Autodesk Inventor part; units mm, degrees
ref_plane "Start Plane" through (0, 0, -4.9897) normal (0, 0, 1) x (1, 0, 0)
ref_plane "End Plane" through (0, 0, 105.0166) normal (0, 0, 1) x (1, 0, 0)
ref_plane "Work Plane4" through (-9.4897, 4.8737, -6.8509) normal (0.4807, -0.2469, -0.8414) x (-0.4571, 0.7483, -0.4807)
ref_plane "Start Plane" through (0, 0, -4.9897) normal (0, 0, 1) x (1, 0, 0)
ref_plane "End Plane" through (0, 0, 105.0166) normal (0, 0, 1) x (1, 0, 0)
sketch "Sketch" plane through (0, 0, 0) normal (0, 0, 1) x (1, 0, 0)
  circle A0 centre (0, 0) radius 6.9342
  circle A1 centre (0, 0) radius 10.668
  dimension "d0" = 21.336
  dimension "d1" = 3.7338
extrude "Body" add sketch "Sketch" along normal up to surface (110.0063 mm away) from surface at -4.9897
sketch "Sketch3" plane through (0, 0, 0) normal (0, 0, 1) x (1, 0, 0)
  line L0 (0, 0) -> (10, 0)
ref_plane "Work Plane3" through (0, 0, 0) normal (0, -1, 0) x (1, 0, 0)
sketch "Sketch4" plane through (0, 0, 0) normal (0, -1, 0) x (1, 0, 0)
  line L0 (-2, -4.9897) -> (12, -4.9897)
  line L1 (-2, 105.0166) -> (12, 105.0166)
  dimension "d7" = 110.0063
ref_plane "Work Plane4" through (-9.4897, 4.8737, -6.8509) normal (0.4807, -0.2469, -0.8414) x (-0.4571, 0.7483, -0.4807)
split "Split1" plane through (-9.4897, 4.8737, -6.8509) removes the side toward (0.4807, -0.2469, -0.8414)
ref_plane "Work Plane5" through (6.4449, 8.5011, -9.0952) normal (-0.392, -0.517, -0.761) x (0.3573, -0.8478, 0.392)
split "Split2" plane through (6.4449, 8.5011, -9.0952) removes the side toward (-0.392, -0.517, -0.761)
ref_plane "Work Plane6" through (-10.5607, 1.5089, 115.9586) normal (0.7772, -0.111, 0.6194) x (0.627, 0.0533, -0.7772)
split "Split3" plane through (-10.5607, 1.5089, 115.9586) removes the side toward (0.7772, -0.111, 0.6194)
ref_plane "Work Plane7" through (0, 10.668, 105.0198) normal (0, -0.2353, 0.9719) x (1, 0, 0)
split "Split4" plane through (0, 10.668, 105.0198) removes the side toward (0, -0.2353, 0.9719)
equation "\"d0\" = G_H"
equation "\"d1\" = G_T"
equation "\"d2\" = G_L"
equation "\"G_H\" = 21.336"
equation "\"G_T\" = 3.7338"
equation "\"G_L\" = 110.00626"
equation "\"G_OFFSET_START\" = 4.98966"
equation "\"G_OFFSET_END\" = 2.57893"
equation "\"d4\" = -G_OFFSET_START"
equation "\"d5\" = G_OFFSET_END + B_L"
equation "\"B_L\" = 102.43767"
properties part number "ANSI - 1/2 x 0.147 - 4.331" material "Steel, Mild"
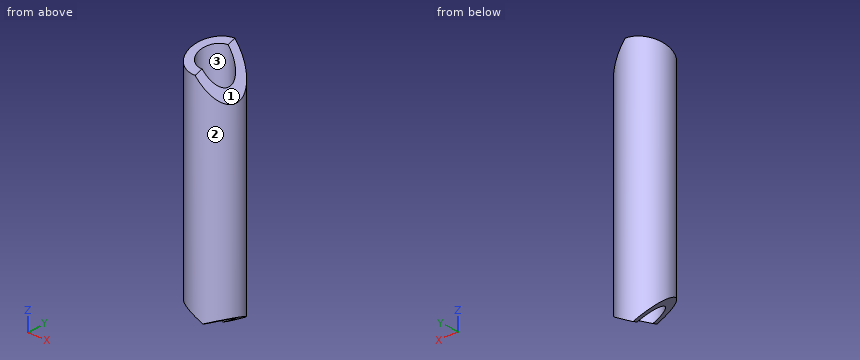
Geometry check sheet. Reference: the model listing, model coordinates, mm. Face numbers are marked on the shaded views. Round coordinates to 2 decimals unless told otherwise and drop trailing zeros. Loops run counter-clockwise (first coordinate to the right, second up) from the corner with the lowest first, then second, coordinate; pieces in that order, holes last.
Item 1: Cross-section at B-B on z = 85. Record the boundary of the cut face in (x, y), then the cut area to 3 significant figures.
Item 2: Cross-section at A-A on y = 2.5. Record the boundary of the cut face in (x, z), then the cut area to 3 significant figures.
Item 3: Cross-section at C-C on y = -5.5. Record the boundary of the cut face in (x, z).
Item 4: Gauge pin test, flat ends, axial feed: pin 1 (4 mm diameter, centred on y = -3, z = 90, fed in from -X); pin 2 (1.5 mm diameter, centred on x = 5, y = -7, fed in from +Z); pin 3 (4 mm diameter, centred on x = 5.5, y = -5.5, fed in from -Z). Record the tip position at first contact, or that the pin passes through.
Item 5: Mould release check, pull along X, two halves, no side actions. Record for the marked faces 1, 2 and 3: pulls with the +X half, pulls with the -X half, needs draft (parallel to the pull), parting line crosses it, or undercut.
Item 6: Thickness scan on line 1 (Y direction, x = 0, z = 59); line 2 (X direction, y = -4.5, z = 79). Record the ranges inside material, lowest first.
Answer sheet:
1. outline: circle Ø21.34 at (0, 0); hole circle Ø13.87 at (0, 0)
1. area: 206 mm2
2. outline: (-10.37, 3.64) - (-6.47, 1.63) - (-6.47, 103.04) - (-10.37, 103.04) - close; (6.47, 2.96) - (10.37, 5.19) - (10.37, 89.87) - (6.47, 94.77) - close
2. area: 736 mm2
3. outline: (-9.14, 8.45) - (-4.22, 5.91) - (-4.22, 101.11) - (-9.14, 101.11) - close; (4.22, 4.03) - (9.14, 6.84) - (9.14, 89.98) - (4.22, 96.15) - close
4. pin 1: stops at x = -10.62
4. pin 2: stops at z = 95.86
4. pin 3: stops at z = 3.78
5. face 1: pulls with the +X half
5. face 2: parting line crosses it
5. face 3: undercut
6. line 1: y = -10.67 to -6.93, 6.93 to 10.67
6. line 2: x = -9.67 to -5.28, 5.28 to 9.67
